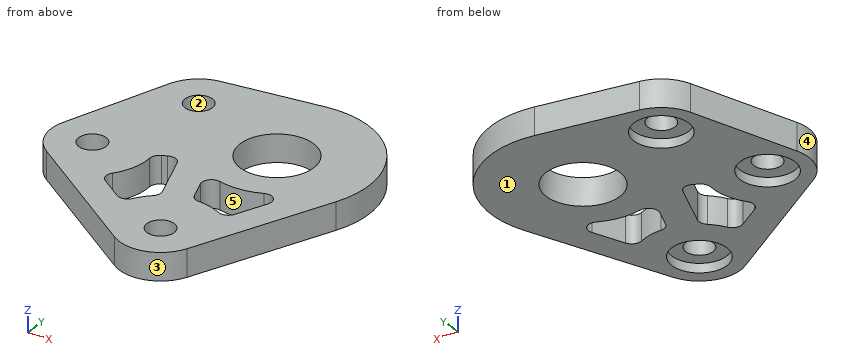
Autodesk Inventor part; units mm, degrees
ref_plane "YZ Plane" through (0, 0, 0) normal (1, 0, 0) x (0, 1, 0)
ref_plane "XZ Plane" through (0, 0, 0) normal (0, 1, 0) x (-1, 0, 0)
ref_plane "XY Plane" through (0, 0, 0) normal (0, 0, 1) x (1, 0, 0)
sketch "スケッチ1" plane through (0, 0, 0) normal (0, 0, 1) x (1, 0, 0)
  circle A0 centre (0, 0) radius 4.025
  line L0 (0, 0) -> (0, -4.025)
  line L1 (0, 0) -> (-1.4816, -16.9353)
  circle A1 centre (-1.4816, -16.9353) radius 1.5
  line L2 (0, 0) -> (-15.4072, -7.1845)
  circle A2 centre (-15.4072, -7.1845) radius 1.5
  line L3 (0, 0) -> (-11.2763, 4.1042)
  circle A3 centre (-11.2763, 4.1042) radius 1.5
  circle A4 centre (0, 0) radius 7.025
  circle A5 centre (0, 0) radius 10.025
  circle A6 centre (-11.2763, 4.1042) radius 4.5
  circle A7 centre (-15.4072, -7.1845) radius 4.5
  circle A8 centre (-1.4816, -16.9353) radius 4.5
  line L4 (-15.5023, 5.6507) -> (-19.6332, -5.6381)
  line L5 (-17.9883, -10.8707) -> (-4.0627, -20.6215)
  line L6 (2.6304, -18.7632) -> (9.1607, -4.072)
  line L7 (-1.2936, 9.9412) -> (-12.3185, 8.5066)
  point P0 (-11.857, 8.5666)
  dimension "d0" = 8.05
  dimension "d1" = 5
  dimension "d2" = 17
  dimension "d3" = 3
  dimension "d4" = 17
  dimension "d5" = 3
  dimension "d6" = 60
  dimension "d7" = 12
  dimension "d8" = 3
  dimension "d9" = 45
  dimension "d12" = 3
  dimension "d18" = 3
  dimension "d19" = 3
  dimension "d20" = 3
  dimension "d21" = 3
extrude "押し出し1" add sketch "スケッチ1" along normal blind 3 contours A0 L3 A4 L1 | L1 A4 L2 A0 | A0 L2 A4 L3 | A4 L3 A6 A5 L1 | L1 A5 L2 A4 | A4 L2 A5 A6 L3 | A5 L6 A8 L1 | L1 A8 L5 A7 L2 A5 | A6 A5 L3 | L3 A5 A6 | L2 A7 L4 A6 A5 | A8 | A5 A6 | A7 | A6 L7 A5
sketch "スケッチ2" plane through (0, 0, 0) normal (0, 0, -1) x (-1, 0, 0)
  circle A0 centre (11.2763, 4.1042) radius 1.5
  circle A1 centre (15.4072, -7.1845) radius 1.5
  circle A2 centre (1.4816, -16.9353) radius 1.5
  circle A3 centre (11.2763, 4.1042) radius 3
  circle A4 centre (15.4072, -7.1845) radius 3
  circle A5 centre (1.4816, -16.9353) radius 3
  point P0 (0, 0)
  dimension "d13" = 6
  dimension "d14" = 6
  dimension "d15" = 6
extrude "押し出し2" cut sketch "スケッチ2" against normal blind 1
sketch "スケッチ3" plane through (0, 0, 0) normal (0, 0, -1) x (-1, 0, 0)
  circle A0 centre (11.2763, 4.1042) radius 3
  circle A1 centre (15.4072, -7.1845) radius 3
  circle A2 centre (1.4816, -16.9353) radius 3
  circle A3 centre (0, 0) radius 4.025
  arc A4 (17.9883, -10.8707) -> (19.6332, -5.6381) centre (15.4072, -7.1845) ccw
  line L0 (15.5023, 5.6507) -> (19.6332, -5.6381)
  arc A5 (15.5023, 5.6507) -> (11.857, 8.5666) centre (11.2763, 4.1042) ccw
  line L1 (1.2936, 9.9412) -> (11.857, 8.5666)
  arc A6 (1.2936, 9.9412) -> (-9.1607, -4.072) centre (0, 0) ccw
  line L2 (-2.6304, -18.7632) -> (-9.1607, -4.072)
  arc A7 (-2.6304, -18.7632) -> (4.0627, -20.6215) centre (1.4816, -16.9353) ccw
  line L3 (17.9883, -10.8707) -> (4.0627, -20.6215)
  arc A8 (0.9065, 6.9663) -> (-6.4194, -2.8535) centre (0, 0) ccw
  line L4 (0.9065, 6.9663) -> (11.4699, 5.5917)
  arc A9 (12.685, 4.6197) -> (11.4699, 5.5917) centre (11.2763, 4.1042) ccw
  line L5 (12.685, 4.6197) -> (16.8159, -6.669)
  arc A10 (16.2676, -8.4132) -> (16.8159, -6.669) centre (15.4072, -7.1845) ccw
  line L6 (16.2676, -8.4132) -> (2.342, -18.164)
  arc A11 (0.111, -17.5446) -> (2.342, -18.164) centre (1.4816, -16.9353) ccw
  line L7 (0.111, -17.5446) -> (-6.4194, -2.8535)
  circle A12 centre (0, 0) radius 7.025
  circle A13 centre (1.4816, -16.9353) radius 6
  circle A14 centre (15.4072, -7.1845) radius 6
  circle A15 centre (11.2763, 4.1042) radius 6
  line L8 (0, 0) -> (15.4072, -7.1845) construction
  line L9 (-0.6339, -1.3595) -> (14.7733, -8.544)
  line L10 (16.0412, -5.825) -> (0.6339, 1.3595)
  arc A16 (0.6339, 1.3595) -> (-0.6339, -1.3595) centre (0, 0) ccw
  arc A17 (14.7733, -8.544) -> (16.0412, -5.825) centre (15.4072, -7.1845) ccw
  line L11 (1.4816, -16.9353) -> (6.3668, -2.9689) construction
  line L12 (2.8975, -17.4306) -> (7.7827, -3.4641)
  line L13 (4.9509, -2.4736) -> (0.0658, -16.4401)
  arc A18 (0.0658, -16.4401) -> (2.8975, -17.4306) centre (1.4816, -16.9353) ccw
  arc A19 (7.7827, -3.4641) -> (4.9509, -2.4736) centre (6.3668, -2.9689) ccw
  point P0 (7.7036, -3.5923)
  point P1 (3.9242, -9.9521)
  point P2 (7.2354, -5.029)
  point P3 (4.8156, -11.9469)
  point P4 (7.1009, -14.8319)
  point P5 (11.5088, -11.7454)
  point P6 (9.5081, -6.0888)
  point P7 (1.9838, -10.9564)
  point P8 (3.735, -5.9498)
  point P9 (-6.4194, -2.8535)
  point P10 (-2.2488, -12.236)
  dimension "d22" = 3
  dimension "d23" = 3
  dimension "d24" = 3
  dimension "d25" = 3
  dimension "d26" = 3
  dimension "d27" = 3
  dimension "d28" = 3
extrude "押し出し3" cut sketch "スケッチ3" against normal blind 10 contours A12 L13 A13 L7 | A14 L6 A13 L12 L9
fillet "フィレット1" radius 1.05 9 edges at (-1.9838, -10.9564, 1.5) (6.4194, -2.8535, 1.5) (2.2488, -12.236, 1.5) (-3.735, -5.9498, 1.5) (-9.5081, -6.0888, 1.5) (-7.2354, -5.029, 1.5) (-4.8156, -11.9469, 1.5) (-7.1009, -14.8319, 1.5) (-11.5088, -11.7454, 1.5)
properties part number "アーム揺動節抑え" material "アルミニウム 2014-T4"
Geometry check sheet. Reference: the model listing, model coordinates, mm. Face numbers are marked on the shaded views. A direction names the side the tool comes from. Round coordinates to 2 decimals unless told otherwise and drop trailing zeros. Order: outer loops, then holes, each group sorted by start corner. A loop starts at its lowest first (then second) coordinate and runs counter-clockwise, first axis right, second up. Notation, with made-up numbers: (-21, 86) -> (11, 86) arc R5 ccw to (11, 91) -> close; hole circle Ø8 at (30.25, 48.5). An arc over 180 degrees is marked (long way). Use one line per item in the form item = value.
1. Go/stop test with flat-tipped pins: pin 1 (1 mm diameter, centred on y = -17, z = 1, fed in from -X); pin 2 (1.5 mm diameter, centred on y = 6.5, z = 2, fed in from +X); pin 3 (1.5 mm diameter, centred on y = -11.5, z = 2.5, fed in from -X). Record where each tip stops, or that it passes through.
Working result:
pin_1 = -9.95
pin_2 = 8.21
pin_3 = -18.15
2. Cross-section at B-B, the plane z = 2.3. Count the separate pieces of the cut face and the enclosed holes in it, plus the area to 3 significant figures.
Working result:
separate_pieces = 1
enclosed_holes = 6
area = 538 mm^2
3. Mould release check, pull along X, two halves, no side actions. Record for the marked faces 1, 2 and 3: pulls with the +X half, pulls with the -X half, needs draft (parallel to the pull), parting line crosses it, or undercut.
Working result:
face_1 = needs draft
face_2 = undercut
face_3 = parting line crosses it
4. Cross-section at A-A, the plane y = 0. Enter the section's corners in (x, z) (3 decimals).
Working result:
outline = (-17.57, 0) -> (-4.025, 0) -> (-4.025, 3) -> (-17.57, 3) -> close; (4.025, 0) -> (10.025, 0) -> (10.025, 3) -> (4.025, 3) -> close
5. Cross-section at C-C, the plane y = 6. Enter the section's corners in (x, z).
Working result:
outline = (-15.36, 0) -> (-13.6, 0) -> (-13.6, 1) -> (-8.95, 1) -> (-8.95, 0) -> (8.03, 0) -> (8.03, 3) -> (-15.36, 3) -> close
6. Scan lines: line 1 along Y through (x, z) = (1, 1.65) (3 decimals); line 2 along X through (y, z) = (-9, 2.6); line 3 along Y through (x, z) = (3, 0.7). Record each from-to range of solid material in increasing order. Write a range as from..to.
Working result:
line_1 = -20.689..-11.473, -6.953..-3.899, 3.899..9.975
line_2 = -19.52..-9.69, -5.85..-2.67, 3.69..6.97
line_3 = -17.93..-10.55, -6.37..-2.68, 2.68..9.57
7. Set-up check for the marked faces 4 and 5: record each of +Z, -Z, +X, -X, +Y, -Y from which the full face is reachable in a straight line by a thin tool's end or side.
Working result:
face_4 = +Z, -Z, -X
face_5 = +Z, -Z
